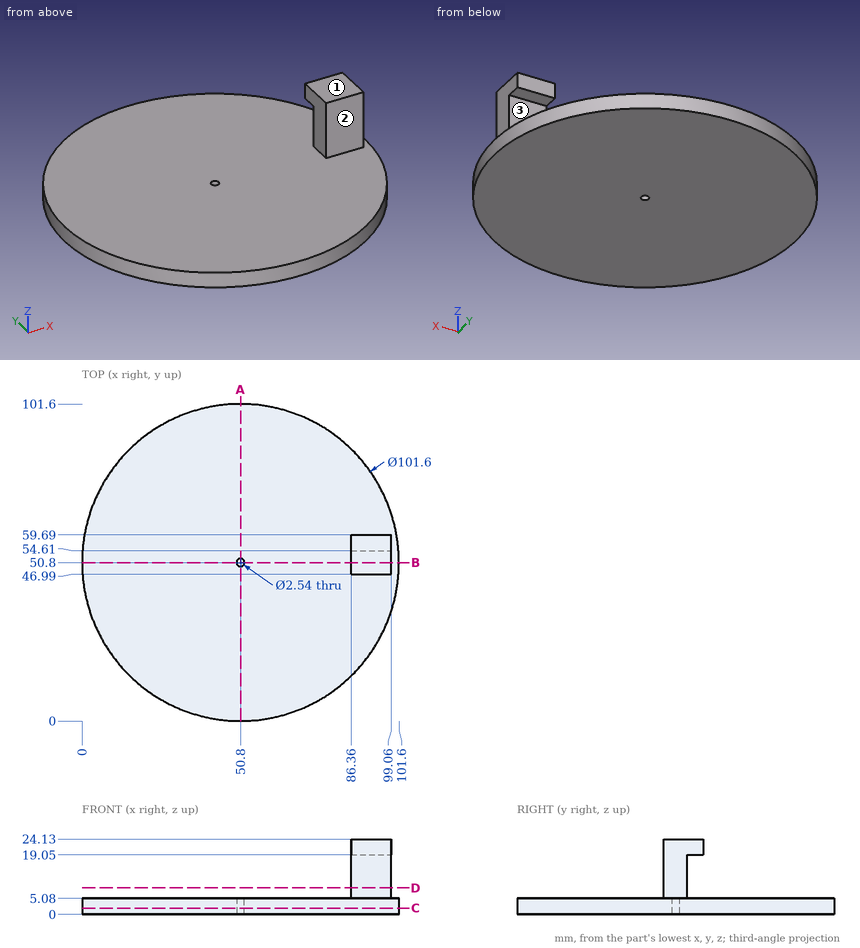
Study the drawing (mm; zero at the part's minimum x, y, z) and answer. Coordinates: 2 decimals unless noted, no trailing zeros. Loops run counter-clockwise (first coordinate to the right, second up) from the corner with the lowest first, then second, coordinate; pieces in that order, holes last. Notation, with made-up numbers: (-28.75, 1) -> (17.25, 1) arc R23 cw to (17.25, 13) -> close; hole circle Ø1 at (74.5, -30.75). An arc over 180 degrees is marked (long way). Write each question's results on one line, items separated by ' | '. Start each with the question number.
1) Find section B-B on y = 50.8. Determine the outline of the cut face in (x, z).
2) The mould has two halves that part along Z. Classify the marked faces 1, 2 and 3: pulls with the +Z half, pulls with the -Z half, needs draft (parallel to the pull), parting line crosses it, or undercut.
3) Consider line 1 along Z through (x, y) = (94, 46); line 2 along Y through (x, z) = (50.8, 3.05); line 3 along Y through (x, z) = (17.5, 3). Determine where each line is inside the solid, lowest interval first.
4) Find section C-C on z = 2. Determine the outline of the cut face in (x, y).
5) Flat-ended cylindrical pins translate along their axes: P1, Ø4, axis at x = 91, z = 13, coming from the +Y side; P2, Ø1.5, axis at y = 63, z = 3.5, coming from the +X side; P3, Ø6.5, axis at x = 95, z = 16, coming from the -Y side. Find the tip coordinate at first contact, or state that the pin passes through.
6) Find section A-A on x = 50.8. Determine the outline of the cut face in (y, z).
7) Find section D-D on z = 8.5. Determine the outline of the cut face in (x, y), then the cut area to 3 significant figures.
Response values:
1) outline: (0, 0) -> (49.53, 0) -> (49.53, 5.08) -> (0, 5.08) -> close; (52.07, 0) -> (101.6, 0) -> (101.6, 5.08) -> (99.06, 5.08) -> (99.06, 24.13) -> (86.36, 24.13) -> (86.36, 5.08) -> (52.07, 5.08) -> close
2) face 1: pulls with the +Z half | face 2: needs draft | face 3: undercut
3) line 1: z = 0 to 5.08 | line 2: y = 0 to 49.53, 52.07 to 101.6 | line 3: y = 12.44 to 89.16
4) outline: circle Ø101.6 at (50.8, 50.8); hole circle Ø2.54 at (50.8, 50.8)
5) P1: stops at y = 54.61 | P2: stops at x = 100.29 | P3: stops at y = 46.99
6) outline: (0, 0) -> (49.53, 0) -> (49.53, 5.08) -> (0, 5.08) -> close; (52.07, 0) -> (101.6, 0) -> (101.6, 5.08) -> (52.07, 5.08) -> close
7) outline: (86.36, 46.99) -> (99.06, 46.99) -> (99.06, 54.61) -> (86.36, 54.61) -> close | area: 96.8 mm^2
